Input: part model. Units: mm. Frame: model coordinates. Face numbers are marked on the shaded views. A direction names the side the tool comes from. Give positions to 0.01 mm unless a question says otherwise; leave off trailing zeros. Loops run counter-clockwise (first coordinate to the right, second up) from the corner with the lowest first, then second, coordinate; pieces in that order, holes last. Notation, with made-up numbers: M 46,86.5 L 86,86.5 A23 ccw 86,123.5 Z; hole C 48,-22.5 d11. An arc over 180 degrees is marked long. Answer as a JSON object with one key per item and string values. Group by question number.
1) Ray query, L1, parallel to Y at x = 0, z = -2.5; L2, parallel to Z at x = 4.5, y = -7.5; L3, parallel to Y at x = 0.7, z = -40. Return the intervals inside material, ascending.
2) Section query B-B on y = 0. Return loops of the section in (x, z), plus the area to 3 significant figures.
3) Section query A-A on x = 0. Return loops of the section in (y, z), plus the area to 3 significant figures.
4) Access query for the marked faces 1, 2, 3, 4 and 5. Directions: +Z, -Z, +X, -X, +Y, -Y. A direction counts if a zero-diameter tool reaches every point of the face in a straight line with its end or side. Return the directions, or none.
5) First-contact query: P1, Ø3, axis at y = 0, z = -30.5, coming from the -X side; P2, Ø1, axis at y = 4.5, z = -36, coming from the +X side; P3, Ø2, axis at y = 2.5, z = 11, coming from the -X side. Flat tips, straight axial feed; report the tip coordinate or a pass-through.
6) Section query C-C on z = -16. Return loops of the section in (x, y).
7) Section query D-D on y = -2.5. Return loops of the section in (x, z), plus the area to 3 significant figures.
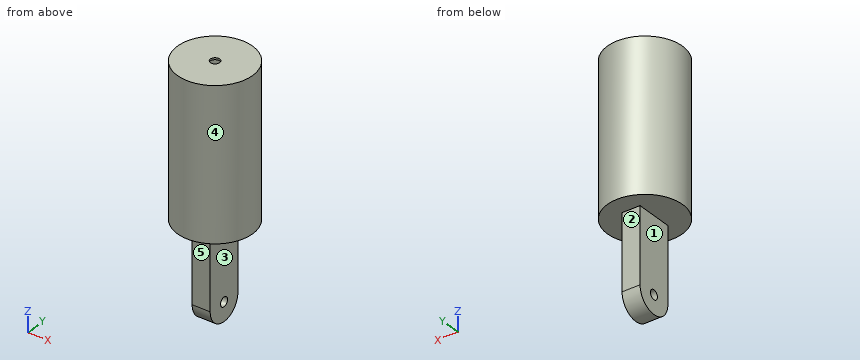
from build123d import *

# Parameters (mm, degrees)
SKETCH1_R           = 10
BOSS_EXTRUDE1_DEPTH = 20
SKETCH3_R           = 9.75
CUT_EXTRUDE1_DEPTH  = 19.5
SKETCH4_R           = 1.25
CUT_EXTRUDE2_DEPTH  = 1
BOSS_EXTRUDE2_DEPTH = 2.4
SKETCH7_R           = 1.25
CUT_EXTRUDE4_DEPTH  = 10


with BuildPart() as part:
    # Sketch1 → Boss-Extrude1 (new, symmetric)
    with BuildSketch(Plane.XY):
        Circle(SKETCH1_R)
    extrude(amount=BOSS_EXTRUDE1_DEPTH, both=True)

    # Sketch3 → Cut-Extrude1 (cut, symmetric)
    with BuildSketch(Plane.XY):
        Circle(SKETCH3_R)
    extrude(amount=CUT_EXTRUDE1_DEPTH, both=True, mode=Mode.SUBTRACT)

    # Sketch4 → Cut-Extrude2 (cut)
    with BuildSketch(Plane.XY.offset(20)):
        Circle(SKETCH4_R)
    extrude(amount=-CUT_EXTRUDE2_DEPTH, mode=Mode.SUBTRACT)

    # Sketch5 → Boss-Extrude2 (add, symmetric)
    with BuildSketch(Plane(origin=(0, 0, 0), x_dir=(0, 0, -1), z_dir=(1, 0, 0))):
        with BuildLine():
            Line((20, 5), (20, -5))
            Line((20, -5), (40, -5))
            ThreePointArc((40, -5), (45, 0), (40, 5))
            Line((40, 5), (20, 5))
        make_face()
    extrude(amount=BOSS_EXTRUDE2_DEPTH, both=True)

    # Sketch7 → Cut-Extrude4 (cut)
    with BuildSketch(Plane(origin=(2.4, 0, 0), x_dir=(0, 0, -1), z_dir=(1, 0, 0))):
        with Locations((40, 0)):
            Circle(SKETCH7_R)
    extrude(amount=-CUT_EXTRUDE4_DEPTH, mode=Mode.SUBTRACT)


solid = part.part
Output:
{
 "1": {"L1": "y = -10 to -9.75, 9.75 to 10", "L2": "z = -20 to -19.5, 19.5 to 20", "L3": "y = -5 to -1.25, 1.25 to 5"},
 "2": {"outline": "M -10,-20 L -2.4,-20 L -2.4,-38.75 L 2.4,-38.75 L 2.4,-20 L 10,-20 L 10,20 L 1.25,20 L 1.25,19.5 L 9.75,19.5 L 9.75,-19.5 L -9.75,-19.5 L -9.75,19.5 L -1.25,19.5 L -1.25,20 L -10,20 Z; M -2.4,-45 L 2.4,-45 L 2.4,-41.25 L -2.4,-41.25 Z", "area": "146 mm^2"},
 "3": {"outline": "M -10,-20 L -5,-20 L -5,-40 A5 ccw 5,-40 L 5,-20 L 10,-20 L 10,20 L 1.25,20 L 1.25,19.5 L 9.75,19.5 L 9.75,-19.5 L -9.75,-19.5 L -9.75,19.5 L -1.25,19.5 L -1.25,20 L -10,20 Z; hole C 0,-40 d2.5", "area": "273 mm^2"},
 "4": {"face 1": "-Z, -X, +Y, -Y", "face 2": "-Z, +X, -X, +Y", "face 3": "-Z, +X, +Y, -Y", "face 4": "+Z, -Z", "face 5": "-Z, +X, -X, -Y"},
 "5": {"P1": "stops at x = -2.4", "P2": "stops at x = 2.4", "P3": "stops at x = -9.89"},
 "6": {"outline": "C 0,0 d20; hole C 0,0 d19.5"},
 "7": {"outline": "M -9.68,-20 L -2.4,-20 L -2.4,-44.33 L 2.4,-44.33 L 2.4,-20 L 9.68,-20 L 9.68,20 L -9.68,20 Z; hole M -9.42,-19.5 L 9.42,-19.5 L 9.42,19.5 L -9.42,19.5 Z", "area": "156 mm^2"}
}
